Read the model definition and answer for the solid it produces. Units are mm, in the model's axes. A direction names the side the tool comes from. Coordinates: 2 decimals unless noted, no trailing zeros. Loops run counter-clockwise (first coordinate to the right, second up) from the corner with the lowest first, then second, coordinate; pieces in that order, holes last.
Autodesk Inventor part; units mm, degrees
ref_plane "YZ Plane" through (0, 0, 0) normal (1, 0, 0) x (0, 1, 0)
ref_plane "XZ Plane" through (0, 0, 0) normal (0, 1, 0) x (-1, 0, 0)
ref_plane "XY Plane" through (0, 0, 0) normal (0, 0, 1) x (1, 0, 0)
sketch "Boceto1" plane through (0, 0, 0) normal (0, 0, 1) x (1, 0, 0)
  line L0 (-4, 8.5) -> (4, 8.5)
  line L1 (4, 8.5) -> (4, -8.5)
  line L2 (4, -8.5) -> (-4, -8.5)
  line L3 (-4, -8.5) -> (-4, 8.5)
  line L4 (0, -11.9) -> (0, 11.9)
  line L5 (-5.6, 0) -> (5.6, 0)
  point P0 (0, 0)
  dimension "d0" = 8
  dimension "d1" = 17
extrude "Extrusión1" add sketch "Boceto1" along normal blind 2
sketch "Boceto2" plane through (0, 0, 2) normal (0, 0, 1) x (1, 0, 0)
  circle A0 centre (0, 5.657) radius 1.25
  circle A1 centre (0, -5.657) radius 1.25
  line L0 (4, 8.5) -> (-4, 8.5)
  line L1 (-4, -8.5) -> (4, -8.5)
  point P0 (0, 0)
  dimension "d4" = 2.5
  dimension "d7" = 2.5
  dimension "d18" = 0
  dimension "d19" = 0
  dimension "d37" = 5.657
  dimension "d38" = 5.657
extrude "Extrusión2" cut sketch "Boceto2" against normal up to surface (2 mm away)
chamfer "Chaflán1" distance 0.5 angle 45 2 edges at (-1.25, 5.657, 2) (-1.25, -5.657, 2)
sketch "Boceto6" plane through (0, 0, 2) normal (0, 0, 1) x (1, 0, 0)
  line L0 (4, 8.5) -> (-4, 8.5)
  line L1 (-4, -8.5) -> (4, -8.5)
  line L2 (-4, 8.5) -> (-2.25, 8.5)
  line L3 (-2.25, 8.5) -> (-2.25, -8.5)
  line L4 (-2.25, -8.5) -> (-4, -8.5)
  line L5 (-4, -8.5) -> (-4, 8.5)
  point P0 (0, 0)
  point P1 (-0.284, 8)
  dimension "d33" = 1.75
extrude "Extrusión6" add sketch "Boceto6" along normal blind 2
sketch "Boceto7" plane through (0, 0, 4) normal (0, 0, 1) x (1, 0, 0)
  line L0 (-4, 8.5) -> (-4, -8.5)
  line L1 (-4, 8.5) -> (-7.5, 8.5)
  line L2 (-7.5, 8.5) -> (-7.5, -8.5)
  line L3 (-7.5, -8.5) -> (-4, -8.5)
  line L4 (-4, -8.5) -> (-4, 8.5)
  line L5 (-9.2, 0) -> (6.2, 0)
  line L6 (-2.25, -8.5) -> (4, -8.5)
  point P0 (0, 0)
  dimension "d39" = 3.5
extrude "Extrusión7" add sketch "Boceto7" against normal up to surface (4 mm away)
sketch "Boceto8" plane through (0, 0, 4) normal (0, 0, 1) x (1, 0, 0)
  line L0 (4, -8.5) -> (4, 8.5)
  line L1 (4, 3) -> (-3, 3)
  line L2 (-3, 3) -> (-3, -3)
  line L3 (-3, -3) -> (4, -3)
  line L4 (4, -3) -> (4, 3)
  line L5 (-9.8, 0) -> (6.3, 0)
  point P0 (0, 0)
  dimension "d43" = 7
  dimension "d44" = 6
extrude "Extrusión8" cut sketch "Boceto8" against normal up to surface (4 mm away)
sketch "Boceto10" plane through (0, 0, 4) normal (0, 0, 1) x (1, 0, 0)
  line L0 (4, 3) -> (-3, 3)
  line L1 (-3, 3) -> (-4.1, 3)
  line L2 (-4.1, 3) -> (-4.1, -3)
  line L3 (-4.1, -3) -> (-3, -3)
  line L4 (-3, -3) -> (-3, 3)
  line L5 (-2.25, -3) -> (-3, -3)
  point P0 (0, 0)
  dimension "d51" = 1.1
extrude "Extrusión10" cut sketch "Boceto10" against normal up to surface (4 mm away)
sketch "Boceto11" plane through (0, 0, 2) normal (0, 0, 1) x (1, 0, 0)
  line L0 (4, 3) -> (4, 8.5)
  line L1 (4, 3) -> (1, 3)
  line L2 (1, 3) -> (1, 2.25)
  line L3 (1, 2.25) -> (4, 2.25)
  line L4 (4, 2.25) -> (4, 3)
  point P0 (0, 0)
  dimension "d54" = 3
  dimension "d55" = 0.75
extrude "Extrusión11" add sketch "Boceto11" against normal up to surface (2 mm away)
mirror "Simetría2" about plane through (0, 0, 0) normal (0, 1, 0) of "Extrusión11"
sketch "Boceto14" plane through (1, 2.25, 2) normal (0, -1, 0) x (1, 0, 0)
  line L0 (3, -2) -> (3, 0)
  line L1 (3, 0) -> (3, 1.0239)
  line L2 (3, -2) -> (-8.5, -2)
  line L3 (3, -2) -> (3, -3.9761)
  line L4 (0.3, -3.5) -> (0.3, 1.5)
  line L5 (3, -3.9761) -> (0.3, -3.5)
  line L6 (3, 1.0239) -> (0.3, 1.5)
  line L7 (3, -3.9761) -> (3, -3.4761)
  line L8 (3, -3.4761) -> (0.3, -3)
  line L9 (3, 1.0239) -> (3, 1.5239)
  line L10 (0.3, 1.5) -> (0.3, 2)
  line L11 (0.3, 2) -> (3, 1.5239)
  line L12 (-8.5, 2) -> (-3.25, 2)
  line L13 (3, 1.5239) -> (3, 2)
  line L14 (3, 2) -> (0.3, 2)
  line L15 (0.3, -3.5) -> (0.3, -4)
  line L16 (0.3, -3.5) -> (0.8, -3.5) construction
  line L17 (0.3, -4) -> (3, -4)
  line L18 (3, -4) -> (3, -3.9761)
  point P0 (-1, -2)
  point P1 (2.8356, -4)
  point P2 (0.3, -2)
  point P3 (-5, -2)
  dimension "d82" = 80
  dimension "d83" = 0.5
  dimension "d84" = 100
  dimension "d85" = 4.5
  dimension "d86" = 0.5
  dimension "d87" = 0.5
  dimension "d93" = 0
  dimension "d94" = 90
  dimension "d95" = 6
  dimension "d96" = 2.7
extrude "Extrusión13" add sketch "Boceto14" along normal up to surface (4.5 mm away) contours L3 L5 L4 L8 | L6 L10 L11 L9 | L18 L17 L15 L5 | L11 L14 L13
sketch "Boceto16" plane through (1.3, -2.25, 4) normal (0, -1, 0) x (1, 0, 0)
  line L0 (0, -0.5) -> (2.7, -0.9761)
  line L1 (2.7, -0.9761) -> (2.7, 0)
  line L2 (2.7, 0) -> (0, 0)
  line L3 (0, 0) -> (0, -0.5)
  line L4 (0, -6) -> (2.7, -6)
  line L5 (2.7, -0.9761) -> (2.7, 0)
  line L6 (0, -6) -> (2.7, -6)
  line L7 (2.7, -6) -> (2.7, 0)
  line L8 (2.7, 0) -> (0, 0)
  line L9 (0, 0) -> (0, -6)
  line L10 (2.7, -6) -> (2.7, -5.4761)
  line L11 (0, -5) -> (0, -6)
  line L12 (2.7, -5.4761) -> (0, -5)
  line L13 (0, 0) -> (0, -0.5)
  point P0 (-1.3, -4)
  point P1 (2.7, -0.9761)
  point P2 (2.7, -6)
  point P3 (2.7, -6)
  point P4 (2.7, -5.4761)
  point P5 (3, -5.529)
extrude "Extrusión15" add sketch "Boceto16" along normal blind 1
mirror "Simetría4" about plane through (0, 0, 0) normal (0, 1, 0) of "Extrusión15"
fillet "Empalme6" radius 0.2 1 edges at (4, 0, -1.4761)
sketch "Boceto18" plane through (0, 0, 4) normal (0, 0, 1) x (1, 0, 0)
  line L0 (-2.25, -8.5) -> (-2.25, -3)
  line L1 (4, 2.25) -> (4, -8.5)
  line L2 (-2.25, -3) -> (4, -3)
  line L3 (4, -3) -> (4, -3.5)
  line L4 (4, -3.5) -> (-2.25, -3.5)
  line L5 (-2.25, -3.5) -> (-2.25, -3)
  line L6 (-2.25, 3) -> (1, 3)
  line L7 (4, 2.25) -> (4, 8.5)
  line L8 (-2.25, 3) -> (4, 3)
  line L9 (4, 3) -> (4, 3.5)
  line L10 (4, 3.5) -> (-2.25, 3.5)
  line L11 (-2.25, 3.5) -> (-2.25, 3)
  point P0 (0, 0)
  point P1 (4, -3.25)
  point P2 (4, 3.25)
  point P3 (-2.25, -3.5)
  point P4 (4, -3)
  point P5 (1, 3)
  point P6 (4, 3)
  point P7 (4, -3)
  dimension "d102" = 0.5
  dimension "d103" = 0.5
extrude "Extrusión16" add sketch "Boceto18" against normal up to surface (2 mm away)
fillet "Empalme7" radius 2 2 edges at (-2.25, -3.5, 3) (-2.25, 3.5, 3)
fillet "Empalme8" radius 1 2 edges at (1, 3, 1) (1, -3, 1)
fillet "Empalme9" radius 4 2 edges at (-2.25, 8.5, 3) (-2.25, -8.5, 3)
sketch "Boceto19" plane through (0, 0, 4) normal (0, 0, 1) x (1, 0, 0)
  line L0 (-4.1, -3) -> (1.3, -3)
  line L1 (-4.1, -3) -> (-4.1, 3)
  line L2 (-4.1, 3) -> (1.3, 3)
  line L3 (1.3, 3) -> (1.3, -3)
  arc A0 (-6.1661, -8.5) -> (-2.222, -5.1667) centre (-6.1661, -4.5) ccw
  arc A1 (-0.25, -3.5) -> (-2.222, -5.1667) centre (-0.25, -5.5) ccw
  line L4 (4, -3.5) -> (-0.25, -3.5)
  line L5 (4, 3.5) -> (4, -3.5)
  line L6 (4, 3.5) -> (-0.25, 3.5)
  arc A2 (-2.222, 5.1667) -> (-0.25, 3.5) centre (-0.25, 5.5) ccw
  arc A3 (-2.222, 5.1667) -> (-6.1661, 8.5) centre (-6.1661, 4.5) ccw
  line L7 (-7.5, 8.5) -> (-7.5, -8.5)
  line L8 (-6.1661, 8.5) -> (-7.5, 8.5)
  line L9 (-7.5, -8.5) -> (-6.1661, -8.5)
  point P0 (0, 0)
extrude "Extrusión17" add sketch "Boceto19" along normal blind 1 contours L1 L2 L3 L0 | L9 L7 L8 A3 A2 L6 L5 L4 A1 A0
sketch "Boceto20" plane through (0, 0, 5) normal (0, 0, 1) x (1, 0, 0)
  line L0 (-7.5, -8.5) -> (-7.5, 8.5)
  line L1 (-7.5, 2.5) -> (-5.5, 2.5)
  line L2 (-5.5, 2.5) -> (-5.5, -2.5)
  line L3 (-5.5, -2.5) -> (-7.5, -2.5)
  line L4 (-7.5, -2.5) -> (-7.5, 2.5)
  line L5 (-9.8, 0) -> (6.3, 0)
  point P0 (0, 0)
  dimension "d111" = 2
  dimension "d112" = 5
extrude "Extrusión18" cut sketch "Boceto20" against normal up to surface (5 mm away)
fillet "Empalme10" radius 1 4 edges at (-7.5, 2.5, 2.5) (-7.5, -2.5, 2.5) (-5.5, 2.5, 2.5) (-5.5, -2.5, 2.5)
equation "\"d4\" = d7"
equation "\"d86\" = d83"
equation "\"d87\" = d86"
properties part number "Soporte Hot End Sensor"
Item 1: A cutting plane is placed at B-B on y = -0.5. Determine the outline of the cut face in (x, z).
Numbers:
outline: (-5.5, 0) - (-4.1, 0) - (-4.1, 4) - (1.3, 4) - (1.3, 3.5) - (4, 3.02) - (4, 5) - (-5.5, 5) - close; (1.3, -2) - (4, -2) - (4, -1.64) arc R0.2 ccw to (3.83, -1.45) - (1.3, -1) - close
Item 2: A cutting plane is placed at D-D on x = -2.75. Determine the outline of the cut face in (y, z), then the cut area to 3 significant figures.
Numbers:
outline: (-8.5, 0) - (-3, 0) - (-3, 4) - (3, 4) - (3, 0) - (8.5, 0) - (8.5, 2) - (6.58, 2) - (6.58, 5) - (-6.58, 5) - (-6.58, 2) - (-8.5, 2) - close
area: 49.5 mm2
Item 3: Which of the six approach directions +Z, -Z, +X, -X, +Y, -Y give full straight-line access (tool end or side, diameter ignored) to faces 1 (the face through (2.67, 0.03, 3.26)), 2 (the face through (0.637, -2.796, 1.014)), 3 (the face through (-5.5, 0, 3))?
Numbers:
face 1: none
face 2: -Z
face 3: +Z, -Z, -X
Item 4: A cutting plane is placed at C-C on z = 0.75. Give the number of separate pieces and of enclosed holes in the cut face, then the cut area to 3 significant figures.
Numbers:
separate pieces: 1
enclosed holes: 2
area: 132 mm2
Item 5: Find the intervals of material crossed by line 1 along Y through (x, z) = (0, 0.5); line 2 along Y through (x, z) = (-3, 1); line 3 along Z through (x, y) = (1, 2.75), in increasing order.
Numbers:
line 1: y = -8.5 to -6.91, -4.41 to -3, 3 to 4.41, 6.91 to 8.5
line 2: y = -8.5 to -3, 3 to 8.5
line 3: z = 0 to 2, 4 to 5
Item 6: A cutting plane is placed at A-A on z = -0.25. Determine the outline of the cut face in (x, y).
Numbers:
outline: (1.3, -3.25) - (4, -3.25) - (4, -2.25) - (1.3, -2.25) - close; (1.3, 2.25) - (4, 2.25) - (4, 3.25) - (1.3, 3.25) - close
Item 7: Given pin 1 (1 mm diameter, centred on y = -0.5, z = -1, fed in from -X); pin 2 (3 mm diameter, centred on x = -1.5, y = 2, fed in from -Z); pin 3 (1.6 mm diameter, centred on x = 3, z = -1.5, fed in from -Y); pin 4 (1.5 mm diameter, centred on x = 0, y = 5.657, fed in from +Z), each flat-ended and moving along its own axis, determine where each tip first touches the part or whether it passes through.
Numbers:
pin 1: stops at x = 1.3
pin 2: stops at z = 0
pin 3: stops at y = -3.25
pin 4: passes through
Item 8: Determine the mould class of faces 4 (the face through (-4.1, 0, 2)), 5 (the face through (-3.554, -7.53, 4.493)), 6 (the face through (1.25, -7.15, 2)), 7 (the face through (-1, 0, 4)) for opening direction Y: released by +Y, released by -Y, zero draft, split by the parting line, or undercut.
Numbers:
face 4: undercut
face 5: released by -Y
face 6: zero draft
face 7: undercut
